from build123d import *

# Parameters (mm, degrees)
SKETCH1_R           = 25.5
SKETCH1_R_2         = 1
BOSS_EXTRUDE1_DEPTH = 1.6
CUT_EXTRUDE1_REACH  = 38.098


with BuildPart() as part:
    # Sketch1 → Boss-Extrude1 (new body)
    with BuildSketch(Plane(origin=(0, 0, 0), x_dir=(1, 0, 0), z_dir=(0, 1, 0))):
        with Locations(Location((0, 0, 0), (0, 0, 270))):
            Circle(SKETCH1_R)
        with Locations(Location((0, 0, 0), (0, 0, 270))):
            Circle(SKETCH1_R_2, mode=Mode.SUBTRACT)
    extrude(amount=BOSS_EXTRUDE1_DEPTH)

    # Sketch2 → Cut-Extrude1 (cut, up to next)
    with BuildSketch(Plane(origin=(0, 1.6, 0), x_dir=(1, 0, 0), z_dir=(0, 1, 0)), mode=Mode.PRIVATE) as cut_extrude1_sk1:
        with BuildLine():
            Line((5.098689446, 11.726182923), (7.398917645, 17.016345603))
            ThreePointArc((7.398917645, 17.016345603), (9.401129193, 18.792276888), (12.049552955, 18.406745328))
            ThreePointArc((12.049552955, 18.406745328), (15.556349186, 15.556349186), (18.406745328, 12.049552955))
            ThreePointArc((18.406745328, 12.049552955), (18.792276888, 9.401129193), (17.016345603, 7.398917645))
            Line((17.016345603, 7.398917645), (11.726182923, 5.098689446))
            ThreePointArc((11.726182923, 5.098689446), (9.663717077, 4.936869827), (7.939396303, 6.079965983))
            ThreePointArc((7.939396303, 6.079965983), (7.071067812, 7.071067812), (6.079965983, 7.939396303))
            ThreePointArc((6.079965983, 7.939396303), (4.936869827, 9.663717077), (5.098689446, 11.726182923))
        make_face()
    cut_extrude1_tool1 = extrude(cut_extrude1_sk1.sketch, amount=-CUT_EXTRUDE1_REACH, mode=Mode.PRIVATE) & part.part
    # Sketch2 → Cut-Extrude1 (cut, up to next)
    with BuildSketch(Plane(origin=(0, 1.6, 0), x_dir=(1, 0, 0), z_dir=(0, 1, 0)), mode=Mode.PRIVATE) as cut_extrude1_sk2:
        with BuildLine():
            Line((-11.726182923, 5.098689446), (-17.016345603, 7.398917645))
            ThreePointArc((-17.016345603, 7.398917645), (-18.792276888, 9.401129193), (-18.406745328, 12.049552955))
            ThreePointArc((-18.406745328, 12.049552955), (-15.556349186, 15.556349186), (-12.049552955, 18.406745328))
            ThreePointArc((-12.049552955, 18.406745328), (-9.401129193, 18.792276888), (-7.398917645, 17.016345603))
            Line((-7.398917645, 17.016345603), (-5.098689446, 11.726182923))
            ThreePointArc((-5.098689446, 11.726182923), (-4.936869827, 9.663717077), (-6.079965983, 7.939396303))
            ThreePointArc((-6.079965983, 7.939396303), (-7.071067812, 7.071067812), (-7.939396303, 6.079965983))
            ThreePointArc((-7.939396303, 6.079965983), (-9.663717077, 4.936869827), (-11.726182923, 5.098689446))
        make_face()
    cut_extrude1_tool2 = extrude(cut_extrude1_sk2.sketch, amount=-CUT_EXTRUDE1_REACH, mode=Mode.PRIVATE) & part.part
    # Sketch2 → Cut-Extrude1 (cut, up to next)
    with BuildSketch(Plane(origin=(0, 1.6, 0), x_dir=(1, 0, 0), z_dir=(0, 1, 0)), mode=Mode.PRIVATE) as cut_extrude1_sk3:
        with BuildLine():
            Line((-11.726182923, -5.098689446), (-17.016345603, -7.398917645))
            ThreePointArc((-17.016345603, -7.398917645), (-18.792276888, -9.401129193), (-18.406745328, -12.049552955))
            ThreePointArc((-18.406745328, -12.049552955), (-15.556349186, -15.556349186), (-12.049552955, -18.406745328))
            ThreePointArc((-12.049552955, -18.406745328), (-9.401129193, -18.792276888), (-7.398917645, -17.016345603))
            Line((-7.398917645, -17.016345603), (-5.098689446, -11.726182923))
            ThreePointArc((-5.098689446, -11.726182923), (-4.936869827, -9.663717077), (-6.079965983, -7.939396303))
            ThreePointArc((-6.079965983, -7.939396303), (-7.071067812, -7.071067812), (-7.939396303, -6.079965983))
            ThreePointArc((-7.939396303, -6.079965983), (-9.663717077, -4.936869827), (-11.726182923, -5.098689446))
        make_face()
    cut_extrude1_tool3 = extrude(cut_extrude1_sk3.sketch, amount=-CUT_EXTRUDE1_REACH, mode=Mode.PRIVATE) & part.part
    # Sketch2 → Cut-Extrude1 (cut, up to next)
    with BuildSketch(Plane(origin=(0, 1.6, 0), x_dir=(1, 0, 0), z_dir=(0, 1, 0)), mode=Mode.PRIVATE) as cut_extrude1_sk4:
        with BuildLine():
            Line((11.726182923, -5.098689446), (17.016345603, -7.398917645))
            ThreePointArc((17.016345603, -7.398917645), (18.792276888, -9.401129193), (18.406745328, -12.049552955))
            ThreePointArc((18.406745328, -12.049552955), (15.556349186, -15.556349186), (12.049552955, -18.406745328))
            ThreePointArc((12.049552955, -18.406745328), (9.401129193, -18.792276888), (7.398917645, -17.016345603))
            Line((7.398917645, -17.016345603), (5.098689446, -11.726182923))
            ThreePointArc((5.098689446, -11.726182923), (4.936869827, -9.663717077), (6.079965983, -7.939396303))
            ThreePointArc((6.079965983, -7.939396303), (7.071067812, -7.071067812), (7.939396303, -6.079965983))
            ThreePointArc((7.939396303, -6.079965983), (9.663717077, -4.936869827), (11.726182923, -5.098689446))
        make_face()
    cut_extrude1_tool4 = extrude(cut_extrude1_sk4.sketch, amount=-CUT_EXTRUDE1_REACH, mode=Mode.PRIVATE) & part.part
    add(cut_extrude1_tool1.solids().sort_by_distance((11.555905, 1.6, -11.555905))[0], mode=Mode.SUBTRACT)
    add(cut_extrude1_tool2.solids().sort_by_distance((-11.555905, 1.6, -11.555905))[0], mode=Mode.SUBTRACT)
    add(cut_extrude1_tool3.solids().sort_by_distance((-11.555905, 1.6, 11.555905))[0], mode=Mode.SUBTRACT)
    add(cut_extrude1_tool4.solids().sort_by_distance((11.555905, 1.6, 11.555905))[0], mode=Mode.SUBTRACT)


solid = part.part
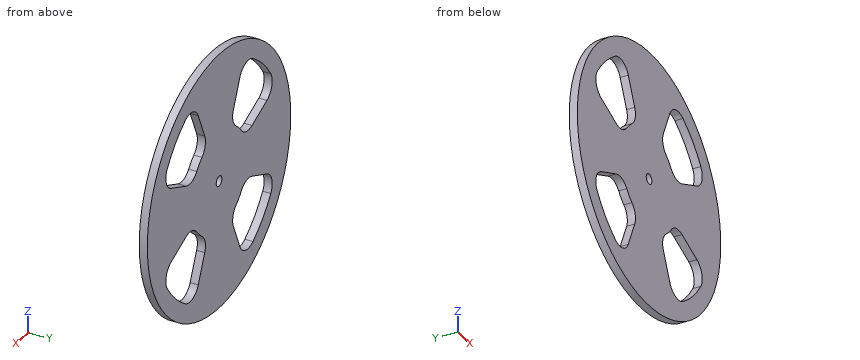
Design review of the part built by this model. Coordinates are the model's own, in mm. Coordinates: 2 decimals unless noted, no trailing zeros. Write each loop counter-clockwise with the first axis right and the second up, starting at its lowest first coordinate (ties: lowest second). Pieces come first, ordered by that corner, then holes. Notation, with made-up numbers: (-28, 24) -> (-4, 24) arc R30 cw to (-4, 60) -> close; hole circle Ø5 at (-23.5, -11). An arc over 180 degrees is marked (long way). Write each question's results on one line, items separated by ' | '. Start each with the question number.
(1) Take a section at D-D on y = 0.3. Give the number of separate pieces and of enclosed holes in the cut face, and give its area (3 significant figures).
(2) Take a section at A-A on z = 0. Write out the cut boundary in (x, y).
(3) Clearance check with a flat-ended pin moving along its axis: P1, Ø1.5, axis at x = 19, z = 5, coming from the -Y side. State where the tip first meets the part, or that it passes through.
(4) Take a section at C-C on z = -13.5. Write out the cut boundary in (x, y).
(5) For line 1 along X through (y, z) = (0.55, 0); line 2 along Z through (x, y) = (16.5, 1.4); line 3 along Z through (x, y) = (18, 1.05), list the stretches that pass through material, from the lowest coordinate up. Write a range as from..to.
(6) Take a section at B-B on x = 0. Write out the cut boundary in (y, z).
Results found:
1) separate pieces: 1 | enclosed holes: 5 | area: 1,500 mm2
2) outline: (-25.5, 0) -> (-1, 0) -> (-1, 1.6) -> (-25.5, 1.6) -> close; (1, 0) -> (25.5, 0) -> (25.5, 1.6) -> (1, 1.6) -> close
3) P1: stops at y = 0
4) outline: (-21.63, 0) -> (-17.37, 0) -> (-17.37, 1.6) -> (-21.63, 1.6) -> close; (-5.87, 0) -> (5.87, 0) -> (5.87, 1.6) -> (-5.87, 1.6) -> close; (17.37, 0) -> (21.63, 0) -> (21.63, 1.6) -> (17.37, 1.6) -> close
5) line 1: x = -25.5..-1, 1..25.5 | line 2: z = -19.44..-14.55, -7.17..7.17, 14.55..19.44 | line 3: z = -18.06..-12.65, -8.07..8.07, 12.65..18.06
6) outline: (0, -25.5) -> (1.6, -25.5) -> (1.6, -1) -> (0, -1) -> close; (0, 1) -> (1.6, 1) -> (1.6, 25.5) -> (0, 25.5) -> close
